Part print with two shaded views. Sizes in mm from the minimum x, y, z corner. A direction names the side the tool comes from. Round coordinates to 2 decimals unless told otherwise and drop trailing zeros. Loops run counter-clockwise (first coordinate to the right, second up) from the corner with the lowest first, then second, coordinate; pieces in that order, holes last. Notation, with made-up numbers: (12, 71) - (47, 71) arc R12 ccw to (47, 83) - close; hole circle Ø5 at (-13.75, 36.25). An arc over 180 degrees is marked (long way). One line per question, with ' | ' between items.
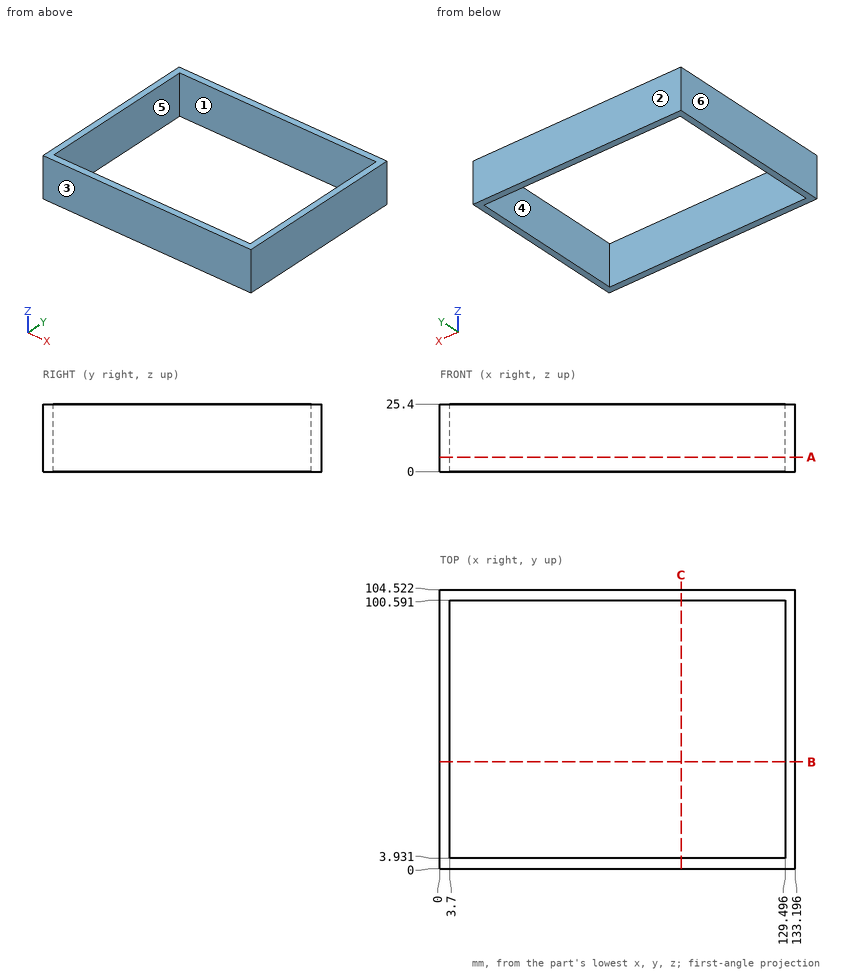
(1) Tool access for the marked faces 1 and 2: list every direction of +Z, -Z, +X, -X, +Y, -Y with a clear straight run to the whole face (end or side of a thin tool).
Results found:
face 1: +Z, -Z | face 2: +Z, -Z, +X, -X, +Y
(2) Cut at C-C, the plane x = 90.5. Write the cut outline in (y, z), then the cut area to 3 significant figures.
Results found:
outline: (0, 0) - (3.93, 0) - (3.93, 25.4) - (0, 25.4) - close; (100.59, 0) - (104.52, 0) - (104.52, 25.4) - (100.59, 25.4) - close | area: 200 mm²
(3) Cut at A-A, the plane z = 5.5. Write the cut outline in (x, y).
Results found:
outline: (0, 0) - (133.2, 0) - (133.2, 104.52) - (0, 104.52) - close; hole (3.7, 3.93) - (129.5, 3.93) - (129.5, 100.59) - (3.7, 100.59) - close
(4) Cut at B-B, the plane y = 40. Write the cut outline in (x, z).
Results found:
outline: (0, 0) - (3.7, 0) - (3.7, 25.4) - (0, 25.4) - close; (129.5, 0) - (133.2, 0) - (133.2, 25.4) - (129.5, 25.4) - close
(5) Two-plate mould, pull along Y, no slides. Class the marked faces 3, 4, 5 and 6: released by +Y, released by -Y, zero draft, split by the parting line, or undercut.
Results found:
face 3: released by -Y | face 4: undercut | face 5: undercut | face 6: zero draft
(6) Probe L1, parallel to X at y = 22.5, z = 14.75; L2, parallel to Y at x = 10, z = 12. List the from-to ranges inside material, lowest first.
Results found:
L1: x = 0 to 3.7, 129.5 to 133.2 | L2: y = 0 to 3.93, 100.59 to 104.52
